Autodesk Inventor part; units mm, degrees
ref_plane "YZ Plane" through (0, 0, 0) normal (1, 0, 0) x (0, 1, 0)
ref_plane "XZ Plane" through (0, 0, 0) normal (0, 1, 0) x (-1, 0, 0)
ref_plane "XY Plane" through (0, 0, 0) normal (0, 0, 1) x (1, 0, 0)
sketch "Skizze1" plane through (0, 0, 0) normal (0, 0, 1) x (1, 0, 0)
  line L0 (8, 0) -> (8, 1.5)
  line L1 (8, 1.5) -> (3.2, 1.5)
  line L2 (3.2, 1.5) -> (2.8933, 1.5)
  line L3 (0, 3) -> (0, 1.1547)
  line L4 (0, 1.1547) -> (1.2, 1.1547)
  line L5 (1.2, 1.1547) -> (1.8667, 0)
  line L6 (1.8667, 0) -> (8, 0)
  line L7 (0, 3) -> (0.2, 3)
  line L8 (0.2, 3) -> (1.7, 1.5)
  line L9 (2.8933, 1.5) -> (1.7, 1.5)
  line L10 (3.2, 1.5) -> (1.7, 1.5) construction
  line L11 (1.7, 1.5) -> (1.7, 1.5)
  line L12 (-12.7, 0) -> (165.1, 0)
  line L13 (0, -1.0566) -> (0, 13.7363)
  dimension "d0" = 8
  dimension "d1" = 4.8
  dimension "d2" = 1.2
  dimension "d3" = 3
  dimension "d6" = 1.7
  dimension "d7" = 45
  dimension "d8" = 2.3094
  dimension "d9" = 60
  dimension "d10" = 6
  dimension "d11" = 3
  dimension "d12" = 0.3067
revolve "Körper" add sketch "Skizze1" angle 360 about axis through (1.8667, 0, 0) along (1, 0, 0) contours L6 L5 L4 L3 L7 L8 L9 L2 L1 L0
sketch "Skizze2" plane through (0, 0, 0) normal (-1, 0, 0) x (0, 0, 1)
  circle A0 centre (0, 0) radius 1.1547
  line L0 (0, -3.6) -> (0, 4.8)
  line L1 (-3.6, 0) -> (4.8, 0)
  line L2 (1.1547, 0) -> (0.5774, -1)
  line L3 (0.5774, -1) -> (-0.5774, -1)
  line L4 (-0.5774, -1) -> (-1.1547, 0)
  line L5 (-1.1547, 0) -> (-0.5774, 1)
  line L6 (-0.5774, 1) -> (0.5774, 1)
  line L7 (0.5774, 1) -> (1.1547, 0)
  point P0 (0, 1.1547)
extrude "Loch" add sketch "Skizze2" against normal up to next contours L7 A0 | A0 L2 | L6 L0 A0 | A0 L0 L3 | L0 L6 A0 | A0 L3 L0 | L4 A0 | A0 L5
thread "Gewinde"
chamfer "Fase1" distance 0.3067 distance2 0.3067 1 edges at (8, -1.5, 0) measured on face at (8, -0.8298, -0.2045)
equation "\"d0\" = NLG"
equation "\"d1\" = GEL"
equation "\"d2\" = INTI"
equation "\"d3\" = GD"
equation "\"d6\" = KOH"
equation "\"d7\" = 0.5 * SEWI"
equation "\"d8\" = 1.1547 * SW"
equation "\"d10\" = KOD"
equation "\"d11\" = BDM"
equation "\"d12\" = GAL"
equation "\"d15\" = GEL"
equation "\"d17\" = -0.5 * SPD + 0.5 * GD"
equation "\"d18\" = GUL"
equation "\"NLG\" = 8"
equation "\"INTI\" = 1.2"
equation "\"GEL\" = 4.8"
equation "\"GAL\" = 0.61345 * TPU"
equation "\"KOH\" = 1.7"
equation "\"KOD\" = 6"
equation "\"GUL\" = 0.61345 * TPU"
equation "\"SPD\" = NND - 1.2269 * TPU"
equation "\"BDM\" = NND"
equation "\"GD\" = NND"
equation "\"SEWI\" = 90deg"
equation "\"SW\" = 2"
equation "\"NND\" = 3"
equation "\"EPV\" = 3.2"
equation "\"E0\" = 1.155 * SW"
equation "\"THREADDIA\" = 3"
equation "\"TPU\" = 0.5"
equation "\"GD1\" = THREADDIA - 1.2269 * TPU"
equation "\"PTC\" = TPU"
equation "\"TOA\" = 30deg"
properties part number "520 209 112"
Part model, mm, in its own coordinate system. A direction names the side the tool comes from. Give positions to 0.01 mm unless a question says otherwise; leave off trailing zeros. Order: outer loops, then holes, each group sorted by start corner. A loop starts at its lowest first (then second) coordinate and runs counter-clockwise, first axis right, second up. Notation, with made-up numbers: M 13.25,3.5 L 35.25,3.5 A25 ccw 35.25,29.5 Z; hole C 7,55.5 d1. An arc over 180 degrees is marked long. Use a Markdown table: item, result. Add a question column.
(1) Saw through at A-A, the plane x = 4. Give the cut face in (y, z), and give its area (3 significant figures).
(2) Drop flat-ended pins along their axis: P1, Ø2, axis at x = 1.5, y = 1.5, coming from the -Z side; P2, Ø0.6, axis at x = 1, z = 0, coming from the -Y side. Give the stop position or say it passes through.
(3) 3-axis set-ups, long thin cutter, end or side, ignore diameter. For faces 1 (the face through (0.64, -0.49, 0.87)), 2 (the face through (0, -1.3, 0)): which of +Z, -Z, +X, -X, +Y, -Y reach the whole face in a straight line?
(4) Mould opens along Y. For faces 3 (the face through (0.64, -0.51, -0.86)), 4 (the face through (4.65, -1.5, -0.07)), 5 (the face through (8, 0, 0)) say: +Y half, -Y half, draft (parallel to the pull), parting line (faces both ways), or undercut.
(5) Probe line 1 along X through (y, z) = (0.2, -0.6); line 2 along Y through (x, z) = (1.25, 0.85) (3 decimals); line 3 along Y through (x, z) = (0.5, -1.3). List the from-to ranges inside material, lowest first. Write a range as [from, to].
Answer key:
| question | item | result |
|---|---|---|
| 1 | outline | C 0,0 d3 |
| 1 | area | 7.07 mm^2 |
| 2 | P1 | z = -2.37 |
| 2 | P2 | y = -2.5 |
| 3 | face 1 | -X |
| 3 | face 2 | +Z, -Z, -X, +Y, -Y |
| 4 | face 3 | undercut |
| 4 | face 4 | parting line |
| 4 | face 5 | draft |
| 5 | line 1 | [1.5, 8] |
| 5 | line 2 | [-1.755, -0.528], [0.528, 1.755] |
| 5 | line 3 | [-2.37, 2.37] |
